Read the model definition and answer for the solid it produces. Units are mm, in the model's axes. Face numbers are marked on the shaded views. A direction names the side the tool comes from. Give positions to 0.01 mm unless a question says otherwise; leave off trailing zeros. Write each loop counter-clockwise with the first axis right and the second up, starting at its lowest first coordinate (ties: lowest second). Pieces come first, ordered by that corner, then holes.
```python
from build123d import *

# Parameters (mm, degrees)
BOSS_EXTRUDE1_REACH      = 123.897
BOSS_EXTRUDE1_END_RADIUS = 31.75
SKETCH2_R                = 12.7
CUT_EXTRUDE1_REACH       = 123.897
CUT_EXTRUDE1_END_RADIUS  = 27.94
SKETCH3_R                = 9.525
BOSS_EXTRUDE2_REACH      = 121.523
BOSS_EXTRUDE2_END_RADIUS = 31.75
SKETCH4_R                = 9.525
CUT_EXTRUDE2_REACH       = 121.523
CUT_EXTRUDE2_END_RADIUS  = 27.94
SKETCH5_R                = 6.35
SKETCH6_R                = 9.525
BOSS_EXTRUDE3_DEPTH      = 6.35
CUT_EXTRUDE3_REACH       = 104.44
SKETCH7_R                = 6.35


with BuildPart() as part:
    # Sketch1 → Revolve1 (revolve)
    with BuildSketch(Plane.XY, mode=Mode.PRIVATE) as revolve1_sk:
        with BuildLine():
            Line((-31.75, 69.85), (-31.75, 19.05))
            ThreePointArc((-31.75, 19.05), (-26.170384182, 5.579615818), (-12.7, 0))
            Line((-12.7, 0), (0, 0))
            Line((0, 0), (0, 3.81))
            Line((0, 3.81), (-12.7, 3.81))
            ThreePointArc((-12.7, 3.81), (-23.476307345, 8.273692655), (-27.94, 19.05))
            Line((-27.94, 19.05), (-27.94, 76.2))
            Line((-27.94, 76.2), (-41.275, 76.2))
            Line((-41.275, 76.2), (-41.275, 69.85))
            Line((-41.275, 69.85), (-31.75, 69.85))
        make_face()
    revolve(revolve1_sk.sketch.rotate(Axis((0, 0, 0), (0, 1, 0)), 270), axis=Axis((0, 0, 0), (0, 1, 0)))

    # Boss-Extrude1: up to this cylinder (the profile starts outside it)
    boss_extrude1_end = Plane(origin=(0, 44.45, 0), z_dir=(0, -1, 0)) * Cylinder(BOSS_EXTRUDE1_END_RADIUS, 312.294, mode=Mode.PRIVATE)
    # Sketch2 → Boss-Extrude1 (add, up to the surface)
    with BuildSketch(Plane(origin=(44.45, 0, 0), x_dir=(0, 0, -1), z_dir=(1, 0, 0)), mode=Mode.PRIVATE) as boss_extrude1_sk1:
        with Locations((0, 44.45)):
            Circle(SKETCH2_R)
    boss_extrude1_tool1 = extrude(boss_extrude1_sk1.sketch, amount=-BOSS_EXTRUDE1_REACH, mode=Mode.PRIVATE) - boss_extrude1_end
    boss_extrude1 = boss_extrude1_tool1.solids().sort_by_distance((44.45, 44.45, 0))[0]
    add(boss_extrude1)

    # Cut-Extrude1: up to this cylinder (the profile starts outside it)
    cut_extrude1_end = Plane(origin=(0, 44.45, 0), z_dir=(0, -1, 0)) * Cylinder(CUT_EXTRUDE1_END_RADIUS, 304.674, mode=Mode.PRIVATE)
    # Sketch3 → Cut-Extrude1 (cut, up to the surface)
    with BuildSketch(Plane(origin=(44.45, 0, 0), x_dir=(0, 0, -1), z_dir=(1, 0, 0)), mode=Mode.PRIVATE) as cut_extrude1_sk1:
        with Locations((0, 44.45)):
            Circle(SKETCH3_R)
    cut_extrude1_tool1 = extrude(cut_extrude1_sk1.sketch, amount=-CUT_EXTRUDE1_REACH, mode=Mode.PRIVATE) - cut_extrude1_end
    cut_extrude1 = cut_extrude1_tool1.solids().sort_by_distance((44.45, 44.45, 0))[0]
    add(cut_extrude1, mode=Mode.SUBTRACT)

    # Mirror3: Boss-Extrude1, Cut-Extrude1 across plane
    add(boss_extrude1.mirror(Plane(origin=(0, 0, 0), x_dir=(0, 0, 1), z_dir=(1, 0, 0))))
    add(cut_extrude1.mirror(Plane(origin=(0, 0, 0), x_dir=(0, 0, 1), z_dir=(1, 0, 0))), mode=Mode.SUBTRACT)

    # Boss-Extrude2: up to this cylinder (the profile starts outside it)
    boss_extrude2_end = Plane(origin=(0, 44.45, 0), z_dir=(0, -1, 0)) * Cylinder(BOSS_EXTRUDE2_END_RADIUS, 307.546, mode=Mode.PRIVATE)
    # Sketch4 → Boss-Extrude2 (add, up to the surface)
    with BuildSketch(Plane.XY.offset(39.37), mode=Mode.PRIVATE) as boss_extrude2_sk1:
        with Locations((0, 44.45)):
            Circle(SKETCH4_R)
    boss_extrude2_tool1 = extrude(boss_extrude2_sk1.sketch, amount=-BOSS_EXTRUDE2_REACH, mode=Mode.PRIVATE) - boss_extrude2_end
    add(boss_extrude2_tool1.solids().sort_by_distance((0, 44.45, 39.37))[0])

    # Cut-Extrude2: up to this cylinder (the profile starts outside it)
    cut_extrude2_end = Plane(origin=(0, 44.45, 0), z_dir=(0, -1, 0)) * Cylinder(CUT_EXTRUDE2_END_RADIUS, 299.926, mode=Mode.PRIVATE)
    # Sketch5 → Cut-Extrude2 (cut, up to the surface)
    with BuildSketch(Plane.XY.offset(39.37), mode=Mode.PRIVATE) as cut_extrude2_sk1:
        with Locations((0, 44.45)):
            Circle(SKETCH5_R)
    cut_extrude2_tool1 = extrude(cut_extrude2_sk1.sketch, amount=-CUT_EXTRUDE2_REACH, mode=Mode.PRIVATE) - cut_extrude2_end
    add(cut_extrude2_tool1.solids().sort_by_distance((0, 44.45, 39.37))[0], mode=Mode.SUBTRACT)

    # Sketch6 → Boss-Extrude3 (add)
    with BuildSketch(Plane.XZ):
        with Locations(Location((0, 0, 0), (0, 0, 90))):
            Circle(SKETCH6_R)
    extrude(amount=BOSS_EXTRUDE3_DEPTH)

    # Sketch7 → Cut-Extrude3 (cut, up to next)
    with BuildSketch(Plane.XZ.offset(6.35), mode=Mode.PRIVATE) as cut_extrude3_sk1:
        with Locations(Location((0, 0, 0), (0, 0, 270))):
            Circle(SKETCH7_R)
    cut_extrude3_tool1 = extrude(cut_extrude3_sk1.sketch, amount=-CUT_EXTRUDE3_REACH, mode=Mode.PRIVATE) & part.part
    add(cut_extrude3_tool1.solids().sort_by_distance((0, -6.35, 0))[0], mode=Mode.SUBTRACT)


solid = part.part
```
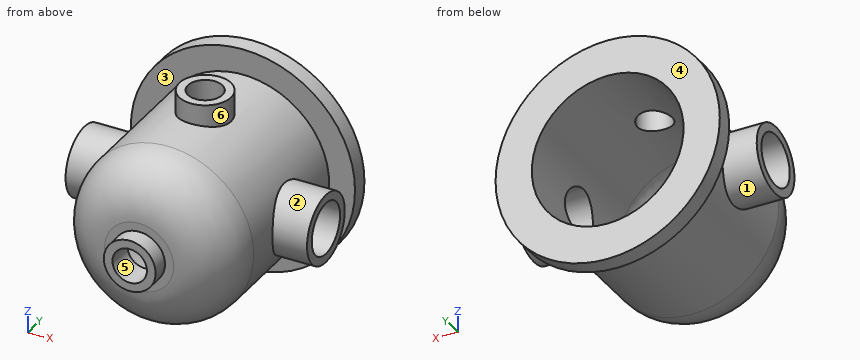
Item 1: Section C-C (z = 0) is taken. Give the number of separate pieces and of enclosed holes in the cut face, and give its area (3 significant figures).
Result set:
separate pieces: 4
enclosed holes: 0
area: 867 mm2
Item 2: Section B-B (x = 38) is taken. Write down the section's boundary in (y, z) (3 decimals).
Result set:
outline: circle Ø25.4 at (44.45, 0); (69.85, -16.113) - (76.2, -16.113) - (76.2, 16.113) - (69.85, 16.113) - close; hole circle Ø19.05 at (44.45, 0)
Item 3: Section A-A (y = 44.45) is taken. Write down the section's boundary in (x, z) (3 decimals).
Result set:
outline: (-44.45, -12.7) - (-29.099, -12.7) arc R31.75 ccw to (29.099, -12.7) - (44.45, -12.7) - (44.45, -9.525) - (26.266, -9.525) arc R27.94 cw to (-26.266, -9.525) - (-44.45, -9.525) - close; (-44.45, 9.525) - (-26.266, 9.525) arc R27.94 cw to (-6.35, 27.209) - (-6.35, 39.37) - (-9.525, 39.37) - (-9.525, 30.288) arc R31.75 ccw to (-29.099, 12.7) - (-44.45, 12.7) - close; (6.35, 27.209) arc R27.94 cw to (26.266, 9.525) - (44.45, 9.525) - (44.45, 12.7) - (29.099, 12.7) arc R31.75 ccw to (9.525, 30.288) - (9.525, 39.37) - (6.35, 39.37) - close
Item 4: Which of the six approach directions +Z, -Z, +X, -X, +Y, -Y give full straight-line access (tool end or side, diameter ignored) to the marked faces 1, 2 and 3?
Result set:
face 1: -X
face 2: +X
face 3: none
Item 5: Determine the mould class of the marked faces 4, 5 and 6 for opening direction Y: pulls with the +Y half, pulls with the -Y half, needs draft (parallel to the pull), parting line crosses it, or undercut.
Result set:
face 4: pulls with the +Y half
face 5: needs draft
face 6: undercut
Item 6: Find the intervals of material crossed by line 1 along Y through (x, z) = (0, 32) (3 decimals); line 2 along Y through (x, z) = (38, -3); line 3 along X through (y, z) = (44, 32), in increasing order.
Result set:
line 1: y = 34.925 to 38.1, 50.8 to 53.975, 69.85 to 76.2
line 2: y = 32.11 to 35.41, 53.49 to 56.79, 69.85 to 76.2
line 3: x = -9.51 to -6.33, 6.33 to 9.51
Item 7: Each of these flat-tipped pins is pushed along its axis until it touches: pin 1 Ø14.5 at (x, z) = (0, 0) entering from +Y; pin 2 Ø3 at (x, y) = (34, 35.5) entering from -Z; pin 3 Ø12 at (x, z) = (21, -7.5) entering from +Y; pin 4 Ø3 at (x, y) = (-19, 17.5) entering from -Z. Where does it stop, or does it pass through?
Result set:
pin 1: stops at y = 3.81
pin 2: stops at z = -10.29
pin 3: stops at y = 76.2
pin 4: stops at z = -26.43
